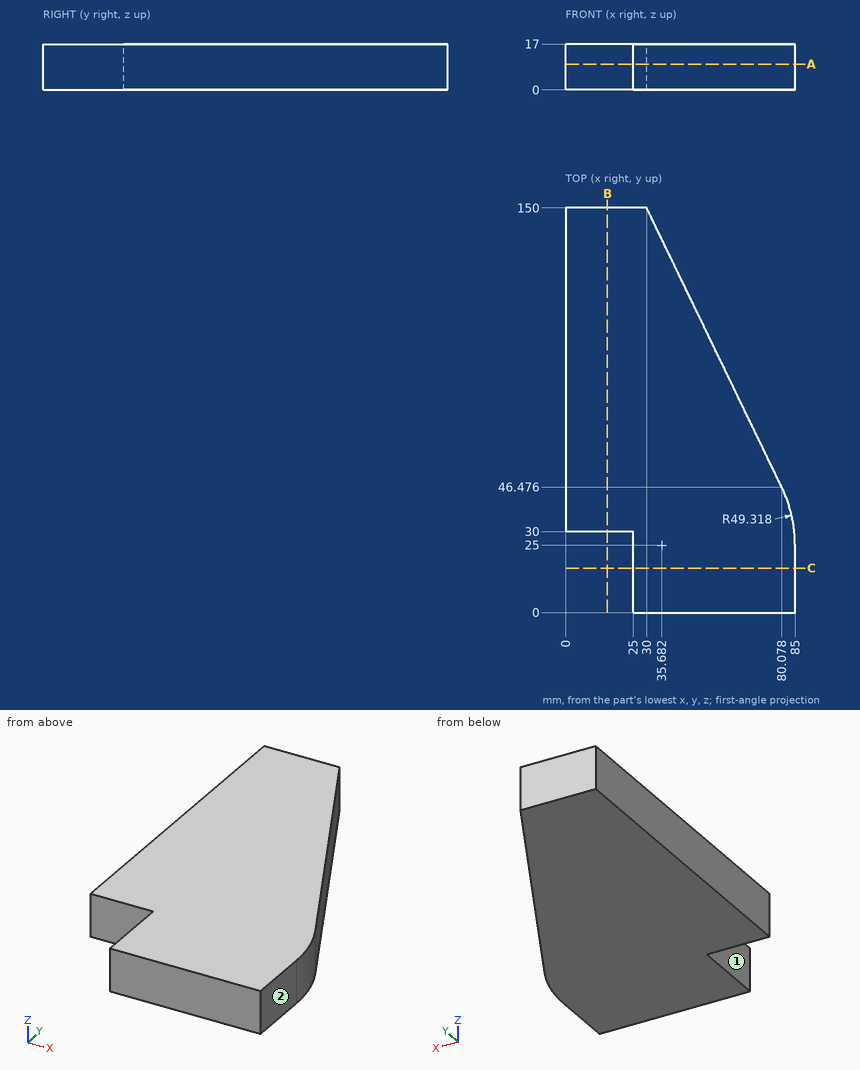
Verification items for this drawing (mm, ordinates from the low corner). A direction names the side the tool comes from. Coordinates: 2 decimals unless noted, no trailing zeros. Order: outer loops, then holes, each group sorted by start corner. A loop starts at its lowest first (then second) coordinate and runs counter-clockwise, first axis right, second up.
Q1. Sectioned sample at C-C on y = 16.5. Record the cut outline in (x, z), and give its area (3 significant figures).
Reply:
outline: (25, 0) - (85, 0) - (85, 17) - (25, 17) - close
area: 1,020 mm2
Q2. Depth check by flat-ended pin: pin 1 Ø1 at (x, z) = (69.5, 6.5) entering from +Y; pin 2 Ø1 at (x, z) = (68, 14) entering from +Y; pin 3 Ø8.5 at (y, z) = (8.5, 11.5) entering from -X. Enter the tip coordinate at first touch or a pass-through.
Reply:
pin 1: stops at y = 69.38
pin 2: stops at y = 72.48
pin 3: stops at x = 25
Q3. Tool access check on the marked faces 1 and 2. Record the directions out of +Z, -Z, +X, -X, +Y, -Y that give a thin tool (end or side, any length) a straight path to the whole face; none if there is none.
Reply:
face 1: +Z, -Z, -X, -Y
face 2: +Z, -Z, +X, +Y, -Y
Q4. Sectioned sample at A-A on z = 9.5. Record the cut outline in (x, y).
Reply:
outline: (0, 30) - (25, 30) - (25, 0) - (85, 0) - (85, 25) arc R49.32 ccw to (80.08, 46.48) - (30, 150) - (0, 150) - close
Q5. Sectioned sample at B-B on x = 15.5. Record the cut outline in (y, z), and give its area (3 significant figures).
Reply:
outline: (30, 0) - (150, 0) - (150, 17) - (30, 17) - close
area: 2,040 mm2
Q6. Thickness scan on probe 1 along X at (y, z) = (10.5, 14.25); probe 2 along Y at (x, z) = (24, 13.5); probe 3 along Y at (x, z) = (42.5, 10.75). Record the ranges inside material, lowest first.
Reply:
probe 1: x = 25 to 85
probe 2: y = 30 to 150
probe 3: y = 0 to 124.16
